Autodesk Inventor part; units mm, degrees
ref_plane "Work Plane1" through (0.75, 6, 0) normal (0, 0, 1) x (1, 0, 0)
ref_plane "YZ Plane" through (0, 0, 0) normal (1, 0, 0) x (0, 1, 0)
ref_plane "XZ Plane" through (0, 0, 0) normal (0, 1, 0) x (-1, 0, 0)
sketch "Sketch1" plane through (0, 0, 0) normal (0, 1, 0) x (-1, 0, 0)
  circle A0 centre (0, 0) radius 4
  circle A1 centre (0, 0) radius 2.5 construction
  line L0 (1.4434, 2.5) -> (2.8868, 0)
  line L1 (2.8868, 0) -> (1.4434, -2.5)
  line L2 (1.4434, -2.5) -> (-1.4434, -2.5)
  line L3 (-1.4434, -2.5) -> (-2.8868, 0)
  line L4 (-2.8868, 0) -> (-1.4434, 2.5)
  line L5 (-1.4434, 2.5) -> (1.4434, 2.5)
  line L6 (0, -2.5) -> (0, -4) construction
  line L7 (0.75, -2.5) -> (0.75, -3.9291)
  line L8 (-0.75, -2.5) -> (-0.75, -3.9291)
  line L9 (2.8868, 0) -> (-2.8868, 0) construction
  line L10 (0.75, 2.5) -> (0.75, 3.9291)
  line L11 (-0.75, 2.5) -> (-0.75, 3.9291)
  point P0 (0, 2.5)
  point P1 (-0.75, 2.5)
  point P2 (-0.75, 3.9291)
  point P3 (0.75, 3.9291)
  point P4 (0.75, 2.5)
  dimension "d1" = 5
  dimension "d0" = 8
  dimension "d2" = 0.75
  dimension "d3" = 0.75
extrude "Extrusion1" add sketch "Sketch1" along normal blind 6 contours A0 L7 L2 L1 L0 L5 L10 | L11 L5 L4 L3 L2 L8 A0
sketch "Sketch2" plane through (0, 0, 0) normal (0, -1, 0) x (1, 0, 0)
  circle A0 centre (0, 0) radius 4.25
  line L0 (2.8868, 0) -> (1.4434, 2.5)
  line L1 (2.8868, 0) -> (1.4434, -2.5)
  line L2 (1.4434, -2.5) -> (-1.4434, -2.5)
  line L3 (-1.4434, -2.5) -> (-2.8868, 0)
  line L4 (-2.8868, 0) -> (-1.4434, 2.5)
  line L5 (-1.4434, 2.5) -> (1.4434, 2.5)
  line L6 (1.4434, 2.5) -> (2.8868, 0)
  dimension "d6" = 8.5
extrude "Extrusion2" add sketch "Sketch2" along normal blind 1
ref_plane "Work Plane1" through (0.75, 6, 0) normal (0, 0, 1) x (1, 0, 0)
sketch "Sketch3" plane through (0.75, 6, 0) normal (0, 0, 1) x (1, 0, 0)
  line L0 (3.25, 0) -> (0, 0)
  line L1 (3.25, 0) -> (3.25, -1)
  line L2 (3.25, -6) -> (3.25, 0)
  line L3 (3.25, -1) -> (3.75, -1)
  line L4 (3.75, -1) -> (3.25, 0)
  line L5 (3.25, 0) -> (2.9426, 0)
  line L6 (2.9426, 0) -> (2.9426, -1)
  line L7 (2.9426, -1) -> (3.25, -1)
  line L8 (-0.75, -6) -> (-0.75, 0) construction
  line L9 (-4.75, 0) -> (-1.5, 0)
  line L10 (-4.75, 0) -> (-4.75, -1)
  line L11 (-4.75, -1) -> (-5.25, -1)
  line L12 (-5.25, -1) -> (-4.75, 0)
  line L13 (-4.4426, 0) -> (-4.4426, -1)
  line L14 (-4.4426, -1) -> (-4.75, -1)
  dimension "d9" = 1
  dimension "d10" = 0.5
revolve "Revolution1" add sketch "Sketch3" angle 35 mid plane about axis through (0, 0, 0) along (0, 1, 0) contours L4 L3 L1 | L10 L11 L12
fillet "Fillet1" radius 0.75 4 edges at (0.75, 0, 3.2145) (-0.75, 0, 3.2145) (0.75, 0, -3.2145) (-0.75, 0, -3.2145)
properties part number "5mmHexInsert"
Could you check a few things on this model? Use its own coordinates, in mm. A direction names the side the tool comes from. Give positions to 0.01 mm unless a question says otherwise; leave off trailing zeros. Write each loop counter-clockwise with the first axis right and the second up, starting at its lowest first coordinate (ties: lowest second). Pieces come first, ordered by that corner, then holes. Notation, with made-up numbers: (17, -8) -> (25, -8) arc R23 ccw to (25, 0) -> close; hole circle Ø10 at (52, -29). An arc over 180 degrees is marked (long way). Write each question's results on one line, items separated by ' | '. Start each with the question number.
Q1. Suppose I cut it at A-A, the plane y = 5.5. List the corners of the cut face in (x, z) for me, and give its area (3 significant figures).
Q2. I need wall thicknesses on probe 1 along Z at (x, y) = (2, 4.5); probe 2 along X at (y, z) = (5, -1.5); probe 3 along Z at (x, y) = (2.75, 3.5). Which ranges of each line are inside material? Lowest first, please.
Q3. Suppose I cut it at B-B, the plane y = -0.5. List the corners of the cut face in (x, z) for me.
Q4. Which directions (+Z, -Z, +X, -X, +Y, -Y) give clear straight access to the entire face, cutting with the end or side of a thin tool? Please do faces 1 (the face through (-2.175, 2.549, 1.233)), 2 (the face through (3.1, 6, 0.1)), 3 (the face through (0.75, 3, 3)).
Q5. I'm going to push flat-ended pins straight in: pin 1 Ø1.1 at (y, z) = (2.5, -3) entering from -X; pin 2 Ø0.8 at (x, z) = (-4.5, -0.5) entering from -Y; pin 3 Ø1.5 at (y, z) = (2, -2.5) entering from +X; pin 4 Ø0.7 at (y, z) = (3, -3.5) entering from +X. Where does each tip first touch, or does it pass through?
Q6. We'd pull the mould along X, two halves only. Please class faces 4 (the face through (1, 2, -2.5)), 5 (the face through (2.285, -0.493, -3.584)), 6 (the face through (-4.253, 5.493, 0.018)): +X half, -X half, draft (parallel to the pull), parting line (faces both ways), or undercut.
Q7. Suppose I cut it at C-C, the plane x = -0.5. List the corners of the cut face in (y, z) for me.
Outcome:
1) outline: (-4.05, -1.28) -> (-3.81, -1.2) arc R4 ccw to (-0.75, -3.93) -> (-0.75, -2.5) -> (-1.44, -2.5) -> (-2.89, 0) -> (-1.44, 2.5) -> (-0.75, 2.5) -> (-0.75, 3.93) arc R4 ccw to (-3.81, 1.2) -> (-4.05, 1.28) arc R4.25 ccw to start; (0.75, -3.93) arc R4 ccw to (3.81, -1.2) -> (4.05, -1.28) arc R4.25 ccw to (4.05, 1.28) -> (3.81, 1.2) arc R4 ccw to (0.75, 3.93) -> (0.75, 2.5) -> (1.44, 2.5) -> (2.89, 0) -> (1.44, -2.5) -> (0.75, -2.5) -> close | area: 25.4 mm2
2) probe 1: -3.46 to -1.54, 1.54 to 3.46 | probe 2: -3.71 to -2.02, 2.02 to 3.71 | probe 3: -2.9 to -0.24, 0.24 to 2.9
3) outline: circle Ø8.5 at (0, 0); hole (-2.89, 0) -> (-1.44, -2.5) -> (1.44, -2.5) -> (2.89, 0) -> (1.44, 2.5) -> (-1.44, 2.5) -> close
4) face 1: +Y, -Y | face 2: +Z, -Z, +X, -X, +Y | face 3: +Z, -Z, +Y
5) pin 1: x = -3.16 | pin 2: y = -1 | pin 3: x = 3.6 | pin 4: x = 2.47
6) face 4: undercut | face 5: parting line | face 6: -X half
7) outline: (-1, -4.22) -> (0, -4.22) -> (0, -3.97) -> (0.19, -3.97) -> (0.19, -2.5) -> (-1, -2.5) -> close; (-1, 2.5) -> (0.19, 2.5) -> (0.19, 3.97) -> (0, 3.97) -> (0, 4.22) -> (-1, 4.22) -> close
